Geometry: see drawing. Coordinates: mm, zero at the bounding-box minimum. A direction names the side the tool comes from. Round coordinates to 2 decimals unless told otherwise and drop trailing zeros. Loops run counter-clockwise (first coordinate to the right, second up) from the corner with the lowest first, then second, coordinate; pieces in that order, holes last.
(1) Mould query, pull axis X, two halves, no side actions, for the marked faces 1, 2 and 3. Classes: pulls with the +X half, pulls with the -X half, needs draft (parallel to the pull), parting line crosses it, or undercut.
(2) Set-up query: the marked faces 4, 5 and 6. Return all of +Z, -Z, +X, -X, +Y, -Y with unobstructed straight access to the full face (end or side cutting, diameter ignored); none if empty.
(3) Section A-A, the plane x = 5.75. Return the cut outline in (y, z).
(4) Material intervals for probe 1 along Y at (x, z) = (5.75, 6.5); probe 2 along X at (y, z) = (5.5, 4); probe 3 along Z at (x, y) = (10, 7.5), sorted ascending.
(5) Section D-D, the plane x = 3. Return the cut outline in (y, z), plus the area to 3 significant figures.
(6) First-contact query: pin 1 Ø5 at (x, y) = (7.5, 3) entering from -Z; pin 2 Ø3 at (y, z) = (2, 3) entering from +X; pin 3 Ø3 at (y, z) = (2, 6) entering from -X; pin 4 Ø5 at (y, z) = (8.5, 5.5) entering from +X. Flat tips, straight axial feed; report the tip coordinate or a pass-through.
(7) Section B-B, the plane z = 6.5. Return the cut outline in (x, y).
(8) Section C-C, the plane y = 7.5. Return the cut outline in (x, z), plus the area to 3 significant figures.
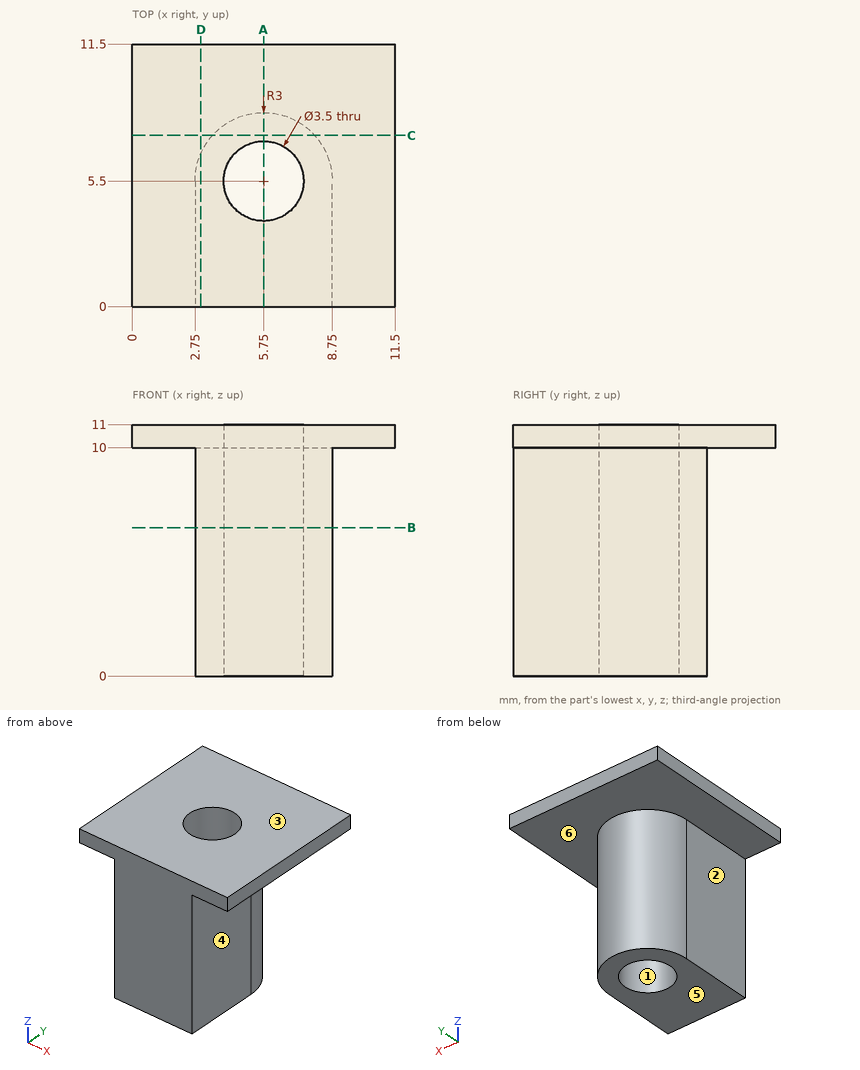
Output values:
1. face 1: undercut
1. face 2: pulls with the -X half
1. face 3: needs draft
2. face 4: -Z, +X, +Y, -Y
2. face 5: -Z, +X, -X, +Y, -Y
2. face 6: -Z, +Y
3. outline: (0, 0) - (3.75, 0) - (3.75, 11) - (0, 11) - close; (7.25, 0) - (8.5, 0) - (8.5, 10) - (11.5, 10) - (11.5, 11) - (7.25, 11) - close
4. probe 1: y = 0 to 3.75, 7.25 to 8.5
4. probe 2: x = 2.75 to 4, 7.5 to 8.75
4. probe 3: z = 10 to 11
5. outline: (0, 0) - (6.7, 0) - (6.7, 10) - (11.5, 10) - (11.5, 11) - (0, 11) - close
5. area: 78.5 mm2
6. pin 1: stops at z = 0
6. pin 2: stops at x = 8.75
6. pin 3: stops at x = 2.75
6. pin 4: stops at x = 8.71
7. outline: (2.75, 0) - (8.75, 0) - (8.75, 5.5) arc R3 ccw to (2.75, 5.5) - close; hole circle Ø3.5 at (5.75, 5.5)
8. outline: (0, 10) - (3.51, 10) - (3.51, 0) - (7.99, 0) - (7.99, 10) - (11.5, 10) - (11.5, 11) - (0, 11) - close
8. area: 56.2 mm2
